```python
from build123d import *

# Parameters (mm, degrees)
F0_W     = 10
F0_H     = 3
F1_DEPTH = 3
F3_SIZE  = 0.4


# Not quite as in the source:
# - a feature of the source that left no trace in its solid (it failed there, or was rolled back) is left out


with BuildPart() as f1:
    # F0 (on Top) → F1 (new body)
    with BuildSketch(Plane.XY):
        Rectangle(F0_W, F0_H)
    extrude(amount=F1_DEPTH)

    # F3
    f3_edges = [f1.edges().sort_by_distance(p)[0] for p in [
        (5, -1.5, 1.5),
        (5, 1.5, 1.5),
        (-5, -1.5, 1.5),
        (-5, 1.5, 1.5),
        (5, 0, 3),
        (-5, 0, 3),
    ]]
    chamfer(f3_edges, length=F3_SIZE)


solid = f1.part
```
Could you check a few things on this model? Use its own coordinates, in mm. Coordinates: 2 decimals unless noted, no trailing zeros. Write each loop counter-clockwise with the first axis right and the second up, starting at its lowest first coordinate (ties: lowest second). Pieces come first, ordered by that corner, then holes. Notation, with made-up numbers: (60.5, -29.5) -> (103.5, -29.5) arc R26 cw to (103.5, 6.5) -> close; hole circle Ø6 at (67, -6.75). An arc over 180 degrees is marked (long way). Write item = value, one per line. Start each with the question number.
(1) We'd pull the mould along X, two halves only. Please class faces 1 (the face through (-5, 0, 1)), 2 (the face through (5, 0, 1)), 3 (the face through (0, -1.5, 1)): released by +X, released by -X, zero draft, split by the parting line, or undercut.
(2) I need wall thicknesses on line 1 (X direction, y = -1.3, z = 1.25). Which ranges of the line are inside material? Lowest first, please. Write a range as [from, to].
(3) Will this pin go through, and if not, where does the flat tip stop? pin 1 (1 mm diameter, centred on x = 2.5, y = 0, fed in from -Z).
(4) I want a section at A-A (z = 2.7). Please give me the cut outline in (x, y), plus the area to 3 significant figures.
Result set:
q1.face_1 = released by -X
q1.face_2 = released by +X
q1.face_3 = zero draft
q2.line_1 = [-4.8, 4.8]
q3.pin_1 = 0
q4.outline = (-4.9, -1.2) -> (-4.6, -1.5) -> (4.6, -1.5) -> (4.9, -1.2) -> (4.9, 1.2) -> (4.6, 1.5) -> (-4.6, 1.5) -> (-4.9, 1.2) -> close
q4.area = 29.2 mm2
